from build123d import *

# Parameters (mm, degrees)
SKETCH2_R           = 5
BOSS_EXTRUDE1_DEPTH = 1.6
SKETCH4_R           = 0.8
CUT_EXTRUDE1_DEPTH  = 32.900742651
FILLET1_R           = 1


with BuildPart() as part:
    # Sketch2 → Boss-Extrude1 (new body)
    # profile 1 of 3: a face of its own
    with BuildSketch(Plane(origin=(0, 0, -5.6), x_dir=(-1, 0, 0), z_dir=(0, 0, -1))):
        with BuildLine():
            Line((-9, -8), (-9, -7.15))
            Line((-9, -7.15), (-23.3, -7.15))
            Line((-23.3, -7.15), (-23.3, 7.15))
            Line((-23.3, 7.15), (-9, 7.15))
            Line((-9, 7.15), (-9, 8))
            ThreePointArc((-9, 8), (-8.95345514, 8.3015349), (-8.818153409, 8.575))
            ThreePointArc((-8.818153409, 8.575), (-9.175329594, 8.262588033), (-9.636306817, 8.15))
            Line((-9.636306817, 8.15), (-24.3, 8.15))
            Line((-24.3, 8.15), (-24.3, -8.15))
            Line((-24.3, -8.15), (-9.636306817, -8.15))
            ThreePointArc((-9.636306817, -8.15), (-9.175329594, -8.262588033), (-8.818153409, -8.575))
            ThreePointArc((-8.818153409, -8.575), (-8.95345514, -8.3015349), (-9, -8))
        make_face()
    # profile 2 of 3: a face of its own
    with BuildSketch(Plane(origin=(0, 0, -5.6), x_dir=(-1, 0, 0), z_dir=(0, 0, -1))):
        with BuildLine():
            Line((-9, 7.15), (-9, -7.15))
            Line((-9, -7.15), (-9, -8))
            ThreePointArc((-9, -8), (-8.95345514, -8.3015349), (-8.818153409, -8.575))
            ThreePointArc((-8.818153409, -8.575), (-8.460977223, -8.887411967), (-8, -9))
            Line((-8, -9), (-2, -9))
            Line((-2, -9), (2, -9))
            Line((2, -9), (8, -9))
            ThreePointArc((8, -9), (8.707106781, -8.707106781), (9, -8))
            Line((9, -8), (9, -2))
            Line((9, -2), (9, 2))
            Line((9, 2), (9, 8))
            ThreePointArc((9, 8), (8.707106781, 8.707106781), (8, 9))
            Line((8, 9), (7.485413277, 9))
            Line((7.485413277, 9), (0.656986152, 9))
            Line((0.656986152, 9), (-2, 9))
            Line((-2, 9), (-8, 9))
            ThreePointArc((-8, 9), (-8.460977223, 8.887411967), (-8.818153409, 8.575))
            ThreePointArc((-8.818153409, 8.575), (-8.95345514, 8.3015349), (-9, 8))
            Line((-9, 8), (-9, 7.15))
        make_face()
        Circle(SKETCH2_R, mode=Mode.SUBTRACT)
    # profile 3 of 3: a face of its own
    with BuildSketch(Plane(origin=(0, 0, -5.6), x_dir=(-1, 0, 0), z_dir=(0, 0, -1))):
        with BuildLine():
            ThreePointArc((1.656986152, 10), (1.364092933, 9.292893219), (0.656986152, 9))
            Line((0.656986152, 9), (7.485413277, 9))
            ThreePointArc((7.485413277, 9), (6.778306496, 9.292893219), (6.485413277, 10))
            Line((6.485413277, 10), (6.485413277, 13.526003096))
            Line((6.485413277, 13.526003096), (7.571199814, 14.611789435))
            Line((7.571199814, 14.611789435), (7.571200029, 16.980216561))
            Line((7.571200029, 16.980216561), (7.4854136, 17.066003006))
            Line((7.4854136, 17.066003006), (7.571200045, 17.151789436))
            Line((7.571200045, 17.151789436), (7.57120026, 19.52021656))
            Line((7.57120026, 19.52021656), (6.485413922, 20.606003096))
            Line((6.485413922, 20.606003096), (1.656986797, 20.606003536))
            Line((1.656986797, 20.606003536), (0.57120026, 19.520217197))
            Line((0.57120026, 19.520217197), (0.571200045, 17.151790072))
            Line((0.571200045, 17.151790072), (0.656986475, 17.066003626))
            Line((0.656986475, 17.066003626), (0.571200029, 16.980217196))
            Line((0.571200029, 16.980217196), (0.571199814, 14.611790072))
            Line((0.571199814, 14.611790072), (1.656986152, 13.526003536))
            Line((1.656986152, 13.526003536), (1.656986152, 10))
        make_face()
        Polygon((1.571199851, 15.026003543), (1.571199991, 16.566003543), (2.071200036, 17.066003498), (1.571200082, 17.566003543), (1.571200223, 19.106003543), (2.071200268, 19.606003498), (6.071200269, 19.606003133), (6.571200223, 19.106003089), (6.571200082, 17.566003089), (6.071200038, 17.066003133), (6.571199991, 16.566003089), (6.571199851, 15.026003089), (6.071199806, 14.526003134), (2.071199805, 14.526003498), align=None, mode=Mode.SUBTRACT)
    extrude(amount=-BOSS_EXTRUDE1_DEPTH)

    # Sketch4 → Cut-Extrude1 (cut, through all)
    with BuildSketch(Plane(origin=(0, 0, -5.6), x_dir=(-1, 0, 0), z_dir=(0, 0, -1))):
        with Locations((-7.5, 7.5)):
            Circle(SKETCH4_R)
        with Locations((-7.5, -7.5)):
            Circle(SKETCH4_R)
        with Locations((7.5, 7.5)):
            Circle(SKETCH4_R)
    extrude(amount=-CUT_EXTRUDE1_DEPTH, mode=Mode.SUBTRACT)

    # Fillet1
    fillet1_edges = [part.edges().sort_by_distance(p)[0] for p in [
        (24.3, -8.15, -4.8),
        (24.3, 8.15, -4.8),
    ]]
    fillet(fillet1_edges, radius=FILLET1_R)


solid = part.part
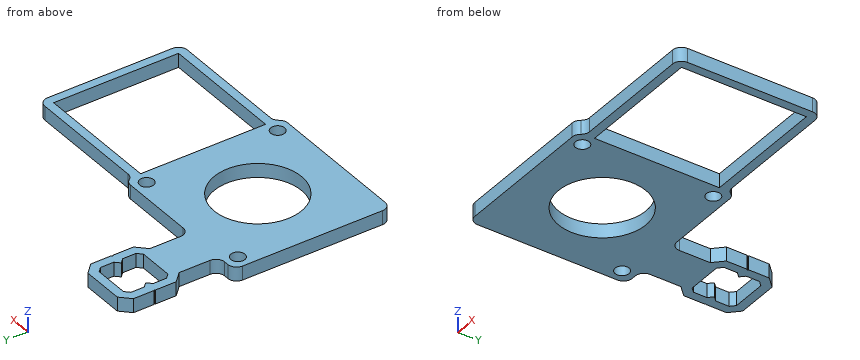
Verification items for the finished model (mm, model axes). Give positions to 0.01 mm unless a question says otherwise; leave off trailing zeros. Loops run counter-clockwise (first coordinate to the right, second up) from the corner with the lowest first, then second, coordinate; pieces in that order, holes last.
1) Depth check by flat-ended pin: pin 1 Ø0.5 at (y, z) = (15.5, -4.5) entering from -X; pin 2 Ø1.5 at (x, y) = (-1, -3) entering from -Z; pin 3 Ø0.5 at (x, z) = (14, -4.5) entering from +Y. Enter the tip coordinate at first touch or a pass-through.
2) Sectioned sample at D-D, the plane y = 0. Enter the section's corners in (x, z), then the cut area to 3 significant figures.
3) Thickness scan on line 1 along X through (y, z) = (0.25, -4.25); line 2 along Y through (x, z) = (7.5, -5.1); line 3 along X through (y, z) = (-5.5, -5.45). Record the ranges inside material, lowest first.
4) Sectioned sample at A-A, the plane y = -5.5. Enter the section's corners in (x, z).
5) Sectioned sample at C-C, the plane x = 7.5. Enter the section's corners in (y, z).
6) Sectioned sample at B-B, the plane x = 19. Enter the section's corners in (y, z), then the cut area to 3 significant figures.
Answers:
1. pin 1: stops at x = -7.57
1. pin 2: passes through
1. pin 3: stops at y = 8.15
2. outline: (-9, -5.6) - (-5, -5.6) - (-5, -4) - (-9, -4) - close; (5, -5.6) - (9, -5.6) - (9, -4) - (5, -4) - close; (23.3, -5.6) - (24.3, -5.6) - (24.3, -4) - (23.3, -4) - close
2. area: 14.4 mm2
3. line 1: x = -9 to -4.99, 4.99 to 9, 23.3 to 24.3
3. line 2: y = -9 to -8.3, -6.7 to 6.7, 8.3 to 9
3. line 3: x = -9 to 9, 23.3 to 24.3
4. outline: (-9, -5.6) - (9, -5.6) - (9, -4) - (-9, -4) - close; (23.3, -5.6) - (24.3, -5.6) - (24.3, -4) - (23.3, -4) - close
5. outline: (-9, -5.6) - (-8.3, -5.6) - (-8.3, -4) - (-9, -4) - close; (-6.7, -5.6) - (6.7, -5.6) - (6.7, -4) - (-6.7, -4) - close; (8.3, -5.6) - (9, -5.6) - (9, -4) - (8.3, -4) - close
6. outline: (-8.15, -5.6) - (-7.15, -5.6) - (-7.15, -4) - (-8.15, -4) - close; (7.15, -5.6) - (8.15, -5.6) - (8.15, -4) - (7.15, -4) - close
6. area: 3.20 mm2
